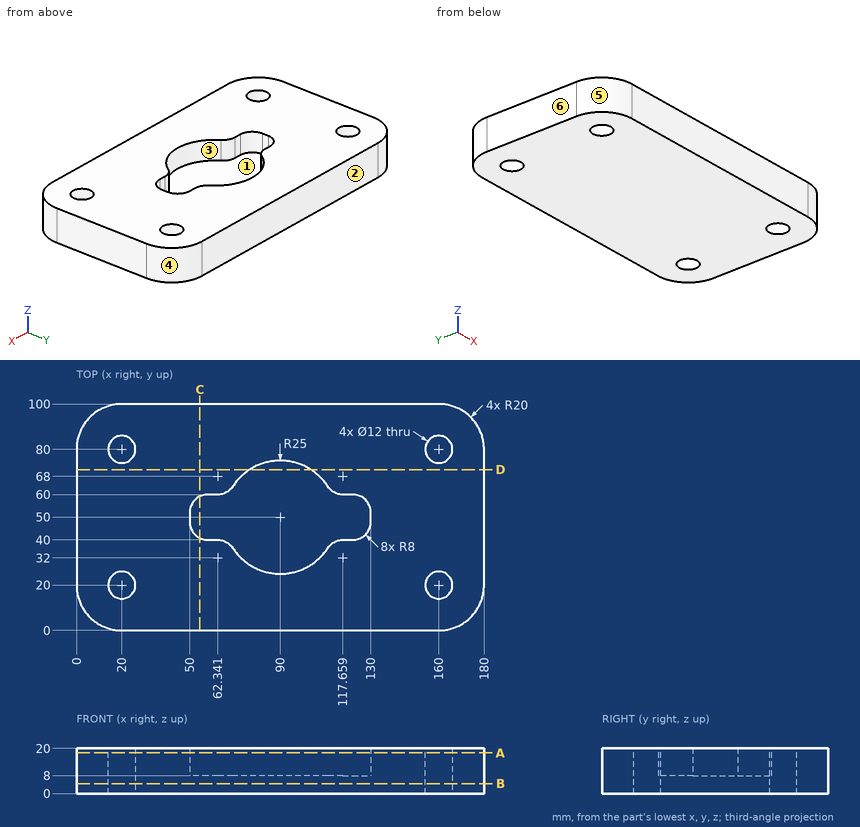
Part print with two shaded views. Sizes in mm from the minimum x, y, z corner. A direction names the side the tool comes from. Give positions to 0.01 mm unless a question says otherwise; leave off trailing zeros. Loops run counter-clockwise (first coordinate to the right, second up) from the corner with the lowest first, then second, coordinate; pieces in that order, holes last. Notation, with made-up numbers: (66, -17.75) -> (79, -17.75) arc R29 ccw to (79, 11.25) -> close; hole circle Ø1 at (-1.75, 49). An arc over 180 degrees is marked (long way). One line per question, with ' | ' between items.
Q1. Cut at B-B, the plane z = 4.5. Write the cut outline in (x, y), plus the area to 3 significant figures.
Filled sheet:
outline: (0, 20) arc R20 ccw to (20, 0) -> (160, 0) arc R20 ccw to (180, 20) -> (180, 80) arc R20 ccw to (160, 100) -> (20, 100) arc R20 ccw to (0, 80) -> close; hole circle Ø12 at (20, 20); hole circle Ø12 at (20, 80); hole circle Ø12 at (160, 20); hole circle Ø12 at (160, 80) | area: 17,200 mm²
Q2. Pull direction Y, two halves, no side cores. Call the marked faces 3, 4, 5 and 6: pulls with the +Y half, pulls with the -Y half, needs draft (parallel to the pull), parting line crosses it, or undercut.
Filled sheet:
face 3: undercut | face 4: pulls with the +Y half | face 5: pulls with the -Y half | face 6: needs draft
Q3. Cut at C-C, the plane x = 54.5. Write the cut outline in (y, z).
Filled sheet:
outline: (0, 0) -> (100, 0) -> (100, 20) -> (59.19, 20) -> (59.19, 8) -> (40.81, 8) -> (40.81, 20) -> (0, 20) -> close
Q4. Drill centre lines: line 1 along Y through (x, z) = (163.5, 9.25) (1 decimal); line 2 along X through (y, z) = (77, 11.25) (1 decimal); line 3 along X through (y, z) = (84, 2.5) (1 decimal). Where is each one in solid material? Low to high. Write a range as [from, to].
Filled sheet:
line 1: y = [0.3, 15.1], [24.9, 75.1], [84.9, 99.7] | line 2: x = [0, 14.8], [25.2, 154.8], [165.2, 180] | line 3: x = [0.4, 15.5], [24.5, 155.5], [164.5, 179.6]
Q5. Drop flat-ended pins along their axis: pin 1 (7 mm diameter, centred on x = 160, y = 20, fed in from -Z); pin 2 (25 mm diameter, centred on x = 91, y = 59, fed in from +Z). Give the stop position or say it passes through.
Filled sheet:
pin 1: passes through | pin 2: stops at z = 8
Q6. Cut at A-A, the plane z = 18. Write the cut outline in (x, y).
Filled sheet:
outline: (0, 20) arc R20 ccw to (20, 0) -> (160, 0) arc R20 ccw to (180, 20) -> (180, 80) arc R20 ccw to (160, 100) -> (20, 100) arc R20 ccw to (0, 80) -> close; hole circle Ø12 at (20, 20); hole circle Ø12 at (20, 80); hole (50, 48) arc R8 ccw to (58, 40) -> (62.34, 40) arc R8 cw to (69.05, 36.36) arc R25 ccw to (110.95, 36.36) arc R8 cw to (117.66, 40) -> (122, 40) arc R8 ccw to (130, 48) -> (130, 52) arc R8 ccw to (122, 60) -> (117.66, 60) arc R8 cw to (110.95, 63.64) arc R25 ccw to (69.05, 63.64) arc R8 cw to (62.34, 60) -> (58, 60) arc R8 ccw to (50, 52) -> close; hole circle Ø12 at (160, 20); hole circle Ø12 at (160, 80)
Q7. Cut at D-D, the plane y = 71. Write the cut outline in (x, z) (1 decimal).
Filled sheet:
outline: (0, 0) -> (180, 0) -> (180, 20) -> (103.6, 20) -> (103.6, 8) -> (76.4, 8) -> (76.4, 20) -> (0, 20) -> close
Q8. Tool access for the marked faces 1 and 2: list every direction of +Z, -Z, +X, -X, +Y, -Y with a clear straight run to the whole face (end or side of a thin tool).
Filled sheet:
face 1: +Z | face 2: +Z, -Z, +X, -X, +Y
